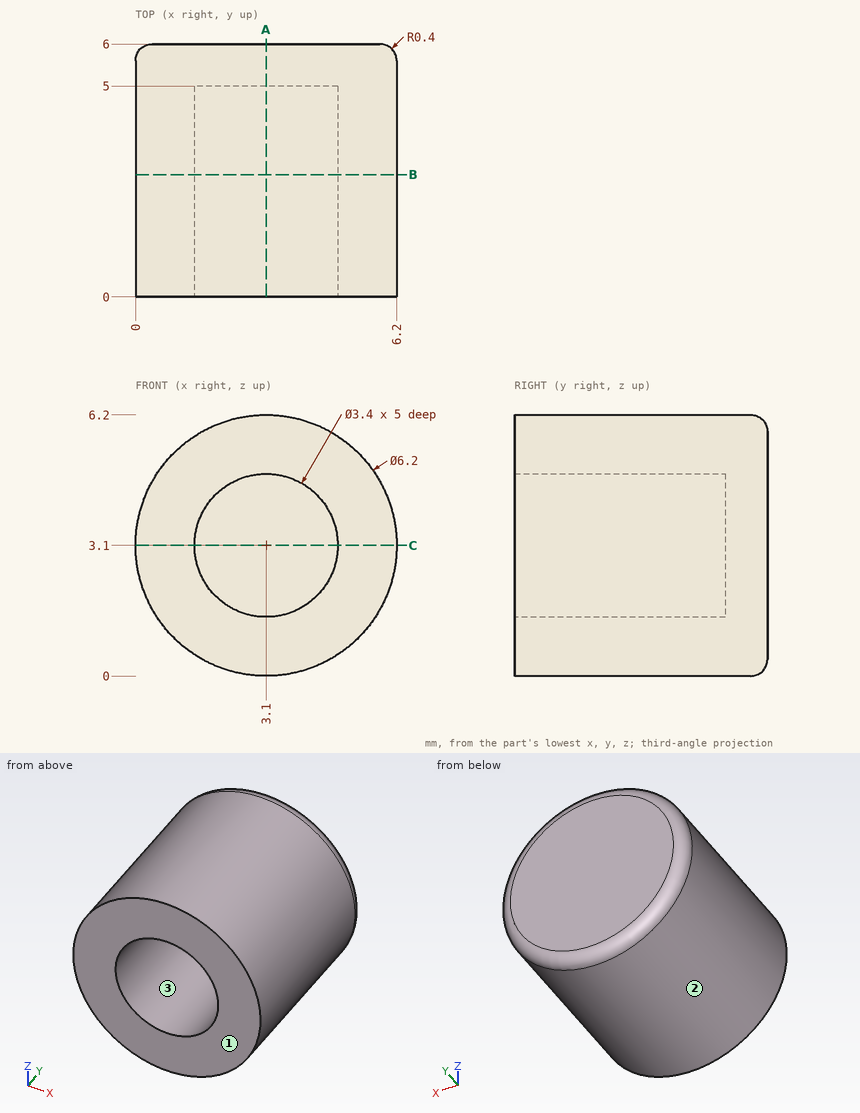
For this review, use the dimensioned drawing (mm, ordinates from the lowest corner) and the shaded views. Coordinates: 2 decimals unless noted, no trailing zeros. Write each loop counter-clockwise with the first axis right and the second up, starting at its lowest first coordinate (ties: lowest second). Pieces come first, ordered by that corner, then holes. Notation, with made-up numbers: (80.25, 11.25) -> (135.25, 11.25) arc R27 ccw to (135.25, 41.25) -> close; hole circle Ø2 at (88.5, 26). An arc over 180 degrees is marked (long way). Put each result on its own line as item: value.
Q1. Take a section at A-A, the plane x = 3.1. State the section outline as (y, z) points, then the cut area to 3 significant figures.
From the geometry:
outline: (0, 0) -> (5.6, 0) arc R0.4 ccw to (6, 0.4) -> (6, 5.8) arc R0.4 ccw to (5.6, 6.2) -> (0, 6.2) -> (0, 4.8) -> (5, 4.8) -> (5, 1.4) -> (0, 1.4) -> close
area: 20.1 mm2
Q2. Wall thickness on L1, parallel to X at y = 2.15, z = 3.1; L2, parallel to Z at x = 4.25, y = 4.55; L3, parallel to Y at x = 3.5, z = 4.25: over which ranges is each line inside the solid? List them lowest first.
From the geometry:
L1: x = 0 to 1.4, 4.8 to 6.2
L2: z = 0.22 to 1.85, 4.35 to 5.98
L3: y = 5 to 6
Q3. Take a section at C-C, the plane z = 3.1. State the section outline as (x, y) points.
From the geometry:
outline: (0, 0) -> (1.4, 0) -> (1.4, 5) -> (4.8, 5) -> (4.8, 0) -> (6.2, 0) -> (6.2, 5.6) arc R0.4 ccw to (5.8, 6) -> (0.4, 6) arc R0.4 ccw to (0, 5.6) -> close
Q4. Clearance check with a flat-ended pin moving along its axis: pin 1 Ø1.5 at (y, z) = (0.5, 4.5) entering from -X. State where the tip first meets the part, or that it passes through.
From the geometry:
pin 1: stops at x = 0.07
Q5. The part is to be moulded in two halves that separate along X. For the marked faces 1, 2 and 3, say which applies: +X half, -X half, draft (parallel to the pull), parting line (faces both ways), or undercut.
From the geometry:
face 1: draft
face 2: parting line
face 3: undercut
Q6. Take a section at B-B, the plane y = 2.9. State the section outline as (x, z) points, then the cut area to 3 significant figures.
From the geometry:
outline: circle Ø6.2 at (3.1, 3.1); hole circle Ø3.4 at (3.1, 3.1)
area: 21.1 mm2
